The model under review builds one solid part; all positions refer to its coordinate system, in mm. Face numbers are marked on the shaded views. A direction names the side the tool comes from. Give positions to 0.01 mm unless a question says otherwise; leave off trailing zeros. Order: outer loops, then holes, each group sorted by start corner. A loop starts at its lowest first (then second) coordinate and runs counter-clockwise, first axis right, second up.
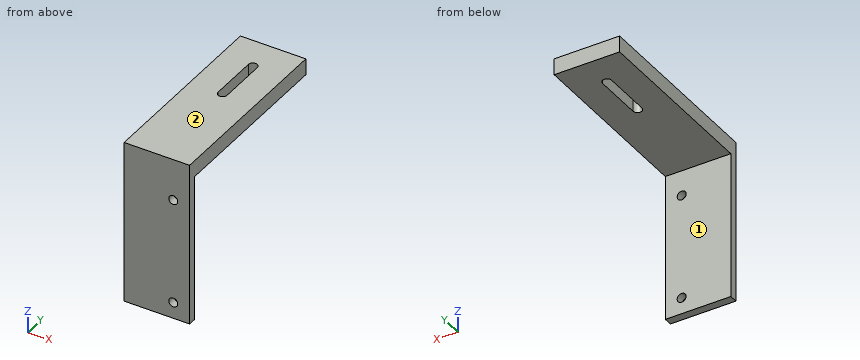
```python
from build123d import *

# Parameters (mm, degrees)
SKETCH_1_W          = 40
SKETCH_1_H          = 5
EXTRUDE_1_DEPTH     = 100
SKETCH_3_R          = 2.75
CUT_EXTRUDE_1_DEPTH = 103.745450916
SKETCH_5_W          = 40
SKETCH_5_H          = 10
EXTRUDE_2_DEPTH     = 110
CUT_EXTRUDE_2_DEPTH = 148.839871767


with BuildPart() as part:
    # 草圖1 → 填料-伸長1 (new body)
    with BuildSketch(Plane.XY):
        with Locations((-3.057052805, 2.5)):
            Rectangle(SKETCH_1_W, SKETCH_1_H)
    extrude(amount=EXTRUDE_1_DEPTH)

    # 草圖3 → 除料-伸長1 (cut, through all)
    with BuildSketch(Plane(origin=(0, 5, 0), x_dir=(1, 0, 0), z_dir=(0, 1, 0))):
        with Locations(Location((6.942947195, -10, 0), (0, 0, 270))):
            Circle(SKETCH_3_R)
        with Locations(Location((6.942947195, -74.5, 0), (0, 0, 270))):
            Circle(SKETCH_3_R)
    extrude(amount=-CUT_EXTRUDE_1_DEPTH, mode=Mode.SUBTRACT)

    # 草圖5 → 填料-伸長2 (add)
    with BuildSketch(Plane(origin=(0, 5, 0), x_dir=(1, 0, 0), z_dir=(0, 1, 0))):
        with Locations((-3.057052805, -95)):
            Rectangle(SKETCH_5_W, SKETCH_5_H)
    extrude(amount=EXTRUDE_2_DEPTH)

    # 草圖7 → 除料-伸長2 (cut, through all)
    with BuildSketch(Plane(origin=(0, 0, 90), x_dir=(-1, 0, 0), z_dir=(0, 0, -1))):
        with BuildLine():
            Line((5.807052805, 95), (5.807052805, 65))
            ThreePointArc((5.807052805, 65), (3.057052805, 62.25), (0.307052805, 65))
            Line((0.307052805, 65), (0.307052805, 95))
            ThreePointArc((0.307052805, 95), (3.057052805, 97.75), (5.807052805, 95))
        make_face()
    extrude(amount=-CUT_EXTRUDE_2_DEPTH, mode=Mode.SUBTRACT)


solid = part.part
```
Item 1: Take a section at D-D (y = 99.5). Give the boundary of the cut face in (x, z).
Values found:
outline: (-23.06, 90) - (16.94, 90) - (16.94, 100) - (-23.06, 100) - close
Item 2: Take a section at A-A (z = 10). Give the boundary of the cut face in (x, y), and give its area (4 significant figures).
Values found:
outline: (-23.06, 0) - (4.19, 0) - (4.19, 5) - (-23.06, 5) - close; (9.69, 0) - (16.94, 0) - (16.94, 5) - (9.69, 5) - close
area: 172.5 mm2
Item 3: For line 1 (X direction, y = 3.75, z = 10); line 2 (Y direction, x = -5, z = 86); line 3 (Z direction, x = -19, y = 70.5), list the stretches that pass through material, from the lowest coordinate up.
Values found:
line 1: x = -23.06 to 4.19, 9.69 to 16.94
line 2: y = 0 to 5
line 3: z = 90 to 100
Item 4: Take a section at C-C (z = 80). Give the boundary of the cut face in (x, y), and give its area (3 significant figures).
Values found:
outline: (-23.06, 0) - (16.94, 0) - (16.94, 5) - (-23.06, 5) - close
area: 200 mm2
Item 5: For the marked faces 1 and 2, list the 3-axis set-ups (+Z, -Z, +X, -X, +Y, -Y) from which the entire face can be reached by the end or side of a thin tool; tool diameter is ignored.
Values found:
face 1: -Z, +X, -X, +Y
face 2: +Z, +X, -X, +Y, -Y
Item 6: Take a section at B-B (x = 1). Give the boundary of the cut face in (y, z), and give its area (3 significant figures).
Values found:
outline: (0, 0) - (5, 0) - (5, 90) - (115, 90) - (115, 100) - (0, 100) - close
area: 1,600 mm2
Item 7: Clearance check with flat-ended pins moving along their axes: pin 1 Ø7 at (x, z) = (6.94, 10) entering from -Y; pin 2 Ø2 at (x, y) = (0.5, 31.5) entering from -Z; pin 3 Ø4 at (x, z) = (-9, 69.5) entering from +Y. State where each tip first meets the part, or that it passes through.
Values found:
pin 1: stops at y = 0
pin 2: stops at z = 90
pin 3: stops at y = 5
